Source: three-view drawing plus pictorial views. Frame: mm from the lowest corner of the part. Give positions to 0.01 mm unless a question says otherwise; leave off trailing zeros. Order: outer loops, then holes, each group sorted by start corner. A loop starts at its lowest first (then second) coordinate and runs counter-clockwise, first axis right, second up.
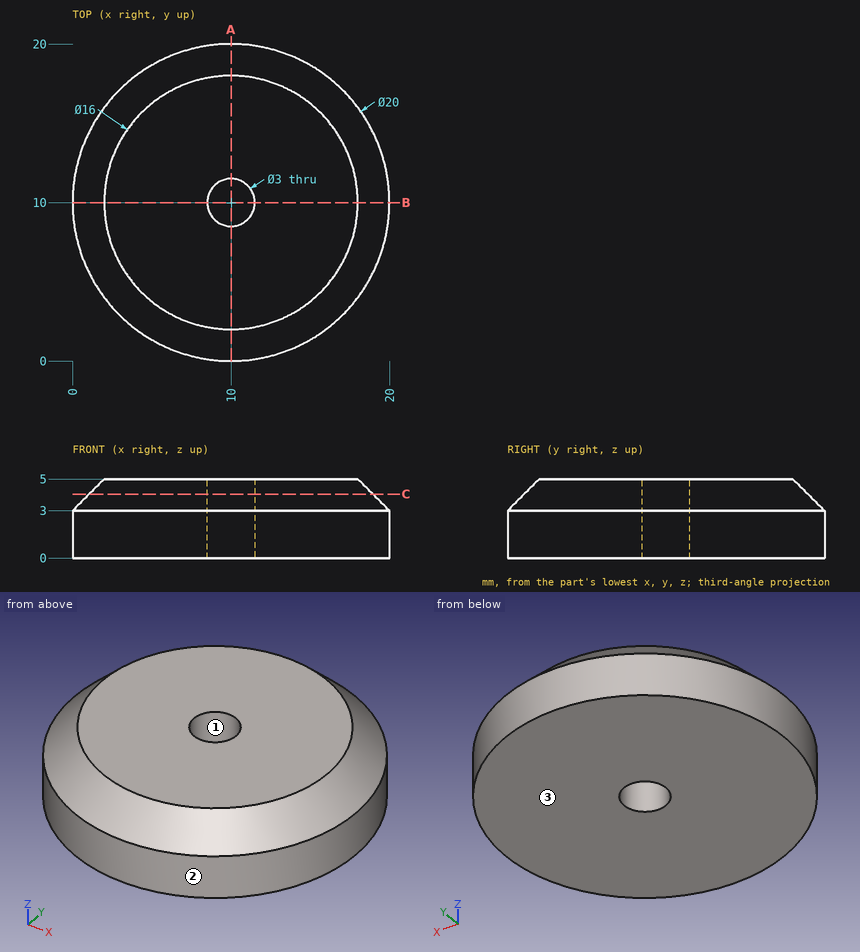
1) Section query A-A on x = 10. Output: boundary loops of the cut face in (y, z), and give its area (3 significant figures).
Checks:
outline: (0, 0) - (8.5, 0) - (8.5, 5) - (2, 5) - (0, 3) - close; (11.5, 0) - (20, 0) - (20, 3) - (18, 5) - (11.5, 5) - close
area: 81.0 mm2
2) Section query C-C on z = 4.05. Output: boundary loops of the cut face in (x, y), and give its area (3 significant figures).
Checks:
outline: circle Ø17.9 at (10, 10); hole circle Ø3 at (10, 10)
area: 245 mm2
3) Pull-direction query (X, two-part tool) for the marked faces 1, 2 and 3; classes: +X half, -X half, draft (parallel to the pull), parting line (faces both ways), or undercut.
Checks:
face 1: undercut
face 2: parting line
face 3: draft
4) First-contact query: pin 1 Ø1.5 at (x, z) = (2.5, 4) entering from +Y; pin 2 Ø1.5 at (x, z) = (11, 2) entering from +Y. Flat tips, straight axial feed; report the tip coordinate or a pass-through.
Checks:
pin 1: stops at y = 16.52
pin 2: stops at y = 20
5) Ray query, L1, parallel to Y at x = 10, z = 1.45; L2, parallel to Y at x = 10, z = 3.15; L3, parallel to Y at x = 2, z = 2.35. Return the intervals inside material, ascending.
Checks:
L1: y = 0 to 8.5, 11.5 to 20
L2: y = 0.15 to 8.5, 11.5 to 19.85
L3: y = 4 to 16
